Study the drawing (mm; zero at the part's minimum x, y, z) and answer. Coordinates: 2 decimals unless noted, no trailing zeros. Loops run counter-clockwise (first coordinate to the right, second up) from the corner with the lowest first, then second, coordinate; pieces in that order, holes last. Notation, with made-up numbers: (-7.75, 21) -> (3.25, 21) arc R24 cw to (3.25, 39) -> close; hole circle Ø3 at (67, 63.5). An arc over 180 degrees is marked (long way). One line per question, with ' | ' between items. Start each with the question number.
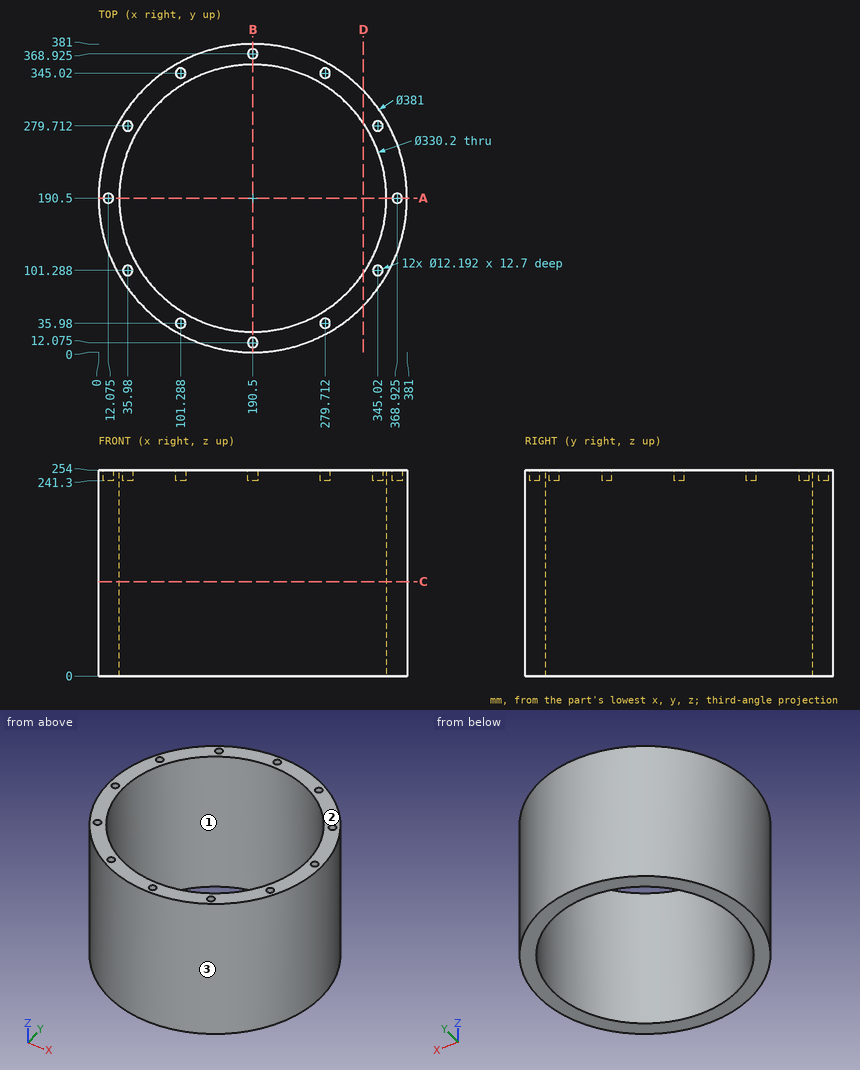
(1) Determine the mould class of the marked faces 1, 2 and 3 for opening direction Y: +Y half, -Y half, draft (parallel to the pull), parting line (faces both ways), or undercut.
(2) Each of these flat-tipped pins is pushed along its axis until it touches: pin 1 Ø6 at (x, y) = (9.5, 192) entering from +Z; pin 2 Ø8 at (x, z) = (214.5, 79) entering from +Y; pin 3 Ø2 at (y, z) = (46.5, 136.5) entering from +X. Where does it stop, or does it pass through?
(3) Section A-A on y = 190.5 is taken. Write down the section's boundary in (x, z), plus the area to 3 significant figures.
(4) Section C-C on z = 116.5 is taken. Write down the section's boundary in (x, y).
(5) Find the intervals of material crossed by probe 1 along X at (y, z) = (190, 251); probe 2 along X at (y, z) = (253, 45) (1 decimal); probe 3 along X at (y, z) = (251, 98.5) (1 decimal), in increasing order. Write a range as from..to.
(6) Section D-D on x = 327 is taken. Write down the section's boundary in (y, z) (1 decimal).
Working result:
1) face 1: undercut | face 2: draft | face 3: parting line
2) pin 1: stops at z = 241.3 | pin 2: stops at y = 379.95 | pin 3: stops at x = 316.36
3) outline: (0, 0) -> (25.4, 0) -> (25.4, 254) -> (18.17, 254) -> (18.17, 241.3) -> (5.98, 241.3) -> (5.98, 254) -> (0, 254) -> close; (355.6, 0) -> (381, 0) -> (381, 254) -> (375.02, 254) -> (375.02, 241.3) -> (362.83, 241.3) -> (362.83, 254) -> (355.6, 254) -> close | area: 12,600 mm2
4) outline: circle Ø381 at (190.5, 190.5); hole circle Ø330.2 at (190.5, 190.5)
5) probe 1: x = 0..6, 18.15..25.4, 355.6..362.85, 375..381 | probe 2: x = 10.5..37.7, 343.3..370.5 | probe 3: x = 9.9..36.9, 344.1..371.1
6) outline: (57.6, 0) -> (97.6, 0) -> (97.6, 254) -> (57.6, 254) -> close; (283.4, 0) -> (323.4, 0) -> (323.4, 254) -> (283.4, 254) -> close
